Can you work these out from the model? Positions are in its coordinate system, mm. A direction names the side the tool comes from. Give positions to 0.01 mm unless a question says otherwise; leave off trailing zeros. Order: outer loops, then holes, each group sorted by start corner. A loop starts at its lowest first (then second) coordinate and runs counter-clockwise, first axis right, second up. Notation, with made-up numbers: M 81.25,79 L 99.25,79 A29 ccw 99.25,118 Z; hole C -32,27.5 d2. An arc over 180 degrees is marked long. Write each question's results on one line, items separated by ' | '.
from build123d import *

# Parameters (mm, degrees)
BOSS_EXTRUDE1_OUTLINE_W   = 50.8
BOSS_EXTRUDE1_OUTLINE_H   = 25.4
BOSS_EXTRUDE1_OUTLINE_W_2 = 45.72
BOSS_EXTRUDE1_OUTLINE_H_2 = 20.32
BOSS_EXTRUDE1_DEPTH       = 711.2
SKETCH3_R                 = 4.166708964
CUT_EXTRUDE1_DEPTH        = 809.244


# Read off the part's stored shape, not the designer's step: Boss-Extrude1
with BuildPart() as part:
    # Boss-Extrude1 outline → Boss-Extrude1 (new body)
    with BuildSketch(Plane(origin=(0, 0, 0), x_dir=(1, 0, 0), z_dir=(0, 1, 0))):
        with Locations((-94.215820821, 5.423243243)):
            Rectangle(BOSS_EXTRUDE1_OUTLINE_W, BOSS_EXTRUDE1_OUTLINE_H)
        with Locations((-94.215820821, 5.423243243)):
            Rectangle(BOSS_EXTRUDE1_OUTLINE_W_2, BOSS_EXTRUDE1_OUTLINE_H_2, mode=Mode.SUBTRACT)
    extrude(amount=BOSS_EXTRUDE1_DEPTH)

    # Sketch3 → Cut-Extrude1 (cut)
    with BuildSketch(Plane(origin=(0, 0, 0), x_dir=(0, 0, -1), z_dir=(1, 0, 0))):
        with Locations(Location((5.423243243, 698.5, 0), (0, 0, 180))):
            Circle(SKETCH3_R)
        with Locations(Location((5.623719473, 673.100791168, 0), (0, 0, 180))):
            Circle(SKETCH3_R)
        with Locations(Location((5.824195703, 647.701582336, 0), (0, 0, 180))):
            Circle(SKETCH3_R)
        with Locations(Location((6.024671933, 622.302373505, 0), (0, 0, 180))):
            Circle(SKETCH3_R)
        with Locations(Location((6.225148163, 596.903164673, 0), (0, 0, 180))):
            Circle(SKETCH3_R)
        with Locations(Location((6.425624393, 571.503955841, 0), (0, 0, 180))):
            Circle(SKETCH3_R)
        with Locations(Location((6.626100623, 546.104747009, 0), (0, 0, 180))):
            Circle(SKETCH3_R)
        with Locations(Location((6.826576853, 520.705538177, 0), (0, 0, 180))):
            Circle(SKETCH3_R)
        with Locations(Location((7.027053082, 495.306329346, 0), (0, 0, 180))):
            Circle(SKETCH3_R)
        with Locations(Location((7.227529312, 469.907120514, 0), (0, 0, 180))):
            Circle(SKETCH3_R)
        with Locations(Location((7.428005542, 444.507911682, 0), (0, 0, 180))):
            Circle(SKETCH3_R)
        with Locations(Location((7.628481772, 419.10870285, 0), (0, 0, 180))):
            Circle(SKETCH3_R)
        with Locations(Location((7.828958002, 393.709494018, 0), (0, 0, 180))):
            Circle(SKETCH3_R)
        with Locations(Location((8.029434232, 368.310285187, 0), (0, 0, 180))):
            Circle(SKETCH3_R)
        with Locations(Location((8.229910462, 342.911076355, 0), (0, 0, 180))):
            Circle(SKETCH3_R)
        with Locations(Location((8.430386692, 317.511867523, 0), (0, 0, 180))):
            Circle(SKETCH3_R)
        with Locations(Location((8.630862922, 292.112658691, 0), (0, 0, 180))):
            Circle(SKETCH3_R)
        with Locations(Location((8.831339152, 266.713449859, 0), (0, 0, 180))):
            Circle(SKETCH3_R)
        with Locations(Location((9.031815381, 241.314241028, 0), (0, 0, 180))):
            Circle(SKETCH3_R)
        with Locations(Location((9.232291611, 215.915032196, 0), (0, 0, 180))):
            Circle(SKETCH3_R)
        with Locations(Location((9.432767841, 190.515823364, 0), (0, 0, 180))):
            Circle(SKETCH3_R)
        with Locations(Location((9.633244071, 165.116614532, 0), (0, 0, 180))):
            Circle(SKETCH3_R)
        with Locations(Location((9.833720301, 139.7174057, 0), (0, 0, 180))):
            Circle(SKETCH3_R)
        with Locations(Location((10.034196531, 114.318196869, 0), (0, 0, 180))):
            Circle(SKETCH3_R)
        with Locations(Location((10.234672761, 88.918988037, 0), (0, 0, 180))):
            Circle(SKETCH3_R)
        with Locations(Location((10.435148991, 63.519779205, 0), (0, 0, 180))):
            Circle(SKETCH3_R)
        with Locations(Location((10.635625221, 38.120570373, 0), (0, 0, 180))):
            Circle(SKETCH3_R)
        with Locations(Location((10.836101451, 12.721361541, 0), (0, 0, 180))):
            Circle(SKETCH3_R)
    extrude(amount=-CUT_EXTRUDE1_DEPTH, mode=Mode.SUBTRACT)


solid = part.part
(1) We'd pull the mould along X, two halves only. Please class faces 1 (the face through (-68.816, 351, -5)), 2 (the face through (-119.616, 351, -5)), 3 (the face through (-117.076, 351, -5)), 4 (the face through (-95, 351, 7.277)): +X half, -X half, draft (parallel to the pull), parting line (faces both ways), or undercut.
Data:
face 1: +X half | face 2: -X half | face 3: undercut | face 4: draft
(2) Imagine slicing it at A-A, the plane x = -105.5. Write out the boundary of the cut face in (y, z), plus the area to 3 significant figures.
Data:
outline: M 0,-18.12 L 711.2,-18.12 L 711.2,-15.58 L 0,-15.58 Z; M 0,4.74 L 711.2,4.74 L 711.2,7.28 L 0,7.28 Z | area: 3,610 mm2
(3) Will this pin go through, and if not, where does the flat tip stop? P1, Ø6.5, axis at y = 698.5, z = -5.42, coming from the -X side.
Data:
P1: passes through
(4) Imagine slicing it at B-B, the plane y = 533. Write out the boundary of the cut face in (x, z).
Data:
outline: M -119.62,-18.12 L -68.82,-18.12 L -68.82,7.28 L -119.62,7.28 Z; hole M -117.08,-15.58 L -71.36,-15.58 L -71.36,4.74 L -117.08,4.74 Z
(5) For faces 5 (the face through (-96, 0, 5)), 6 (the face through (-95, 351, -15.583)), which set-ups out of +Z, -Z, +X, -X, +Y, -Y let a thin tool reach every point of the face, with its end or its side?
Data:
face 5: +Z, -Z, +X, -X, -Y | face 6: +Y, -Y
(6) I need wall thicknesses on L1, parallel to X at y = 141, z = -5.25; L2, parallel to Z at x = -97, y = 268.5. Which ranges of each line are inside material? Lowest first, please. Write a range as from..to.
Data:
L1: x = -119.62..-117.08, -71.36..-68.82 | L2: z = -18.12..-15.58, 4.74..7.28
